```python
from build123d import *

# Parameters (mm, degrees)
SKETCH_1_R          = 50
SKETCH_1_R_2        = 32
EXTRUDE_1_DEPTH     = 15
SKETCH_2_R          = 2.5
CUT_EXTRUDE_1_DEPTH = 15
SKETCH_3_R          = 30
CUT_EXTRUDE_2_DEPTH = 15
FILLET_1_R          = 4


with BuildPart() as part:
    # 草图1 → 凸台-拉伸1 (new body)
    with BuildSketch(Plane(origin=(0, 0, 0), x_dir=(1, 0, 0), z_dir=(0, 1, 0))):
        with Locations(Location((0, 0, 0), (0, 0, 270))):
            Circle(SKETCH_1_R)
        with Locations(Location((0, 0, 0), (0, 0, 270))):
            Circle(SKETCH_1_R_2, mode=Mode.SUBTRACT)
    extrude(amount=EXTRUDE_1_DEPTH)

    # 草图2 → 切除-拉伸1 (cut)
    with BuildSketch(Plane(origin=(0, 15, 0), x_dir=(1, 0, 0), z_dir=(0, 1, 0))):
        with Locations(Location((38.5, 0, 0), (0, 0, 270))):
            Circle(SKETCH_2_R)
        with Locations(Location((-38.5, 0, 0), (0, 0, 90))):
            Circle(SKETCH_2_R)
        with Locations(Location((0, 38.5, 0), (0, 0, 270))):
            Circle(SKETCH_2_R)
        with Locations(Location((0, -38.5, 0), (0, 0, 90))):
            Circle(SKETCH_2_R)
    extrude(amount=-CUT_EXTRUDE_1_DEPTH, mode=Mode.SUBTRACT)

    # 草图3 → 切除-拉伸2 (cut)
    with BuildSketch(Plane(origin=(0, 15, 0), x_dir=(1, 0, 0), z_dir=(0, 1, 0))):
        with BuildLine():
            ThreePointArc((-39.480519481, -6.425619157), (-28.284271247, -28.284271247), (-6.425619157, -39.480519481))
            ThreePointArc((-6.425619157, -39.480519481), (0, -32), (6.425619157, -39.480519481))
            ThreePointArc((6.425619157, -39.480519481), (28.284271247, -28.284271247), (39.480519481, -6.425619157))
            ThreePointArc((39.480519481, -6.425619157), (32, 0), (39.480519481, 6.425619157))
            ThreePointArc((39.480519481, 6.425619157), (28.284271247, 28.284271247), (6.425619157, 39.480519481))
            ThreePointArc((6.425619157, 39.480519481), (0, 32), (-6.425619157, 39.480519481))
            ThreePointArc((-6.425619157, 39.480519481), (-28.284271247, 28.284271247), (-39.480519481, 6.425619157))
            ThreePointArc((-39.480519481, 6.425619157), (-32, 0), (-39.480519481, -6.425619157))
        make_face()
        Circle(SKETCH_3_R, mode=Mode.SUBTRACT)
    extrude(amount=-CUT_EXTRUDE_2_DEPTH, mode=Mode.SUBTRACT)

    # 圆角1
    fillet_1_edges = [part.edges().sort_by_distance(p)[0] for p in [
        (39.480519481, 7.5, 6.425619157),
        (6.425619157, 7.5, 39.480519481),
        (-6.425619157, 7.5, 39.480519481),
        (-39.480519481, 7.5, 6.425619157),
        (-39.480519481, 7.5, -6.425619157),
        (-6.425619157, 7.5, -39.480519481),
        (6.425619157, 7.5, -39.480519481),
        (39.480519481, 7.5, -6.425619157),
    ]]
    fillet(fillet_1_edges, radius=FILLET_1_R)


solid = part.part
```
For this review, take the finished solid that the model builds, in its own axes (mm). A direction names the side the tool comes from. Round coordinates to 2 decimals unless told otherwise and drop trailing zeros. Write each loop counter-clockwise with the first axis right and the second up, starting at its lowest first coordinate (ties: lowest second). Pieces come first, ordered by that corner, then holes. Notation, with made-up numbers: (54, 24.5) -> (99, 24.5) arc R19 cw to (99, 37.5) -> close; hole circle Ø4 at (47, 33). An arc over 180 degrees is marked (long way). One line per question, with ' | ' between items. Start each with the question number.
(1) Add section C-C, the plane x = -14. Write out the cut boundary in (y, z), plus the area to 3 significant figures.
(2) Add section D-D, the plane z = -21.5. Write out the cut boundary in (x, y).
(3) Tool access review of faces 1 (the face through (-28.486, 7.605, 28.081)), 2 (the face through (34, 15, 0)): name each direction out of +Z, -Z, +X, -X, +Y, -Y from which nothing blocks a thin tool from reaching the whole face with its end or side.
(4) Add section A-A, the plane z = 0. Write out the cut boundary in (x, y), plus the area to 3 significant figures.
(5) Insertion check: P1, Ø8, axis at x = -14.5, y = 12, coming from the +Z side; P2, Ø6, axis at x = -38.5, z = 0, coming from the +Y side; P3, Ø6, axis at y = 7.5, z = -25.5, coming from the +X side; P4, Ø4, axis at x = 0, z = 38.5, coming from the +Y side. Each pin has a flat end and moves straight along its axis. Give the tip position at first contact, or say it passes through.
(6) Add section B-B, the plane x = 0. Write out the cut boundary in (y, z), plus the area to 3 significant figures.
(7) For line 1 along Z through (x, y) = (35, 5.5); line 2 along Z through (x, y) = (-19, 6.75); line 3 along Z through (x, y) = (-8, 11.75), list the stretches that pass through material, from the lowest coordinate up. Write a range as from..to.
(8) Mouldability with a two-part tool opening along Z and no side actions: class faces 3 (the face through (36.06, 7.6, -0.54)), 4 (the face through (34, 0, 0)), 5 (the face through (15.02, 7.4, 47.69)) as released by +Z, released by -Z, zero draft, split by the parting line, or undercut.
Answer list:
1) outline: (0, -48) -> (15, -48) -> (15, -37.47) -> (0, -37.47) -> close; (0, 37.47) -> (15, 37.47) -> (15, 48) -> (0, 48) -> close | area: 316 mm²
2) outline: (-45.14, 0) -> (-33.73, 0) -> (-33.73, 15) -> (-45.14, 15) -> close; (33.73, 0) -> (45.14, 0) -> (45.14, 15) -> (33.73, 15) -> close
3) face 1: +Y, -Y | face 2: +Z, -Z, +X, -X, +Y
4) outline: (-50, 0) -> (-41, 0) -> (-41, 15) -> (-50, 15) -> close; (-36, 0) -> (-32, 0) -> (-32, 15) -> (-36, 15) -> close; (32, 0) -> (36, 0) -> (36, 15) -> (32, 15) -> close; (41, 0) -> (50, 0) -> (50, 15) -> (41, 15) -> close | area: 390 mm²
5) P1: z = 48.89 | P2: y = 15 | P3: x = 44.65 | P4: through
6) outline: (0, -50) -> (15, -50) -> (15, -41) -> (0, -41) -> close; (0, -36) -> (15, -36) -> (15, -32) -> (0, -32) -> close; (0, 32) -> (15, 32) -> (15, 36) -> (0, 36) -> close; (0, 41) -> (15, 41) -> (15, 50) -> (0, 50) -> close | area: 390 mm²
7) line 1: -35.71..-19.36, -5.48..5.48, 19.36..35.71 | line 2: -46.25..-35.2, 35.2..46.25 | line 3: -49.36..-38.24, 38.24..49.36
8) face 3: undercut | face 4: zero draft | face 5: split by the parting line
